```python
from build123d import *

# Parameters (mm, degrees)
SKETCH1_W   = 2.7
SKETCH1_H   = 10.5
SKETCH1_H_2 = 10.579195959
PANEL_DEPTH = 2.7


with BuildPart() as part:
    # Sketch1 → Panel (new body)
    with BuildSketch(Plane(origin=(0, 0, 0), x_dir=(0, 0, -1), z_dir=(1, 0, 0))):
        Polygon((3.2125, 30.5), (83.4125, 30.5), (94.9125, 30.5), (94.9125, -12.68), (86.975, -12.68), (6.775, -12.68), (-1.1625, -12.68), (-1.1625, 30.5), align=None)
        with Locations((8.125, 15.172642531)):
            Rectangle(SKETCH1_W, SKETCH1_H, mode=Mode.SUBTRACT)
        with Locations((85.625, 15.212240511)):
            Rectangle(SKETCH1_W, SKETCH1_H_2, mode=Mode.SUBTRACT)
        with Locations((28.125, 15.212240511)):
            Rectangle(SKETCH1_W, SKETCH1_H_2, mode=Mode.SUBTRACT)
    extrude(amount=PANEL_DEPTH)


solid = part.part
```
Check sheet for the modelled part. Datum: model origin and axes. Units: mm. A direction names the side the tool comes from. Round coordinates to 2 decimals unless told otherwise and drop trailing zeros. Write each loop counter-clockwise with the first axis right and the second up, starting at its lowest first coordinate (ties: lowest second). Pieces come first, ordered by that corner, then holes. Notation, with made-up numbers: M -11,54.5 L 46,54.5 A26 ccw 46,87.5 Z; hole C 81.5,84 d7. An arc over 180 degrees is marked long. Write item = value, one per line. Start each with the question number.
1. Scan lines: line 1 (Z direction, x = 2.4, y = 14) (1 decimal); line 2 (Y direction, x = 0.3, z = -84.5). Record each from-to range of solid material in increasing order. Write a range as [from, to].
2. Gauge pin test, flat end, axial feed: pin 1 (1 mm diameter, centred on y = 17.5, z = -69.5, fed in from -X). Record the tip position at first contact, or that the pin passes through.
3. Section check B-B, the plane z = -8. Record the cut outline in (x, y).
4. Tool access check on faces 1 (the flat face through (1, 9.923, -28)), 2 (the flat face through (1, 30.5, -48)). Record the directions out of +Z, -Z, +X, -X, +Y, -Y that give a thin tool (end or side, any length) a straight path to the whole face; none if there is none.
5. Release check for a two-part mould opening along Z. For faces 3 (the flat face through (2.7, 9, -48)), 4 (the flat face through (1, 20.423, -8)), 5 (the flat face through (1, 9, 1.162)) record: pulls with the +Z half, pulls with the -Z half, needs draft (parallel to the pull), parting line crosses it, or undercut.
6. Section check A-A, the plane y = 14. Record the cut outline in (x, z) (1 decimal), then the cut area to 3 significant figures.
7. Section check C-C, the plane x = 0.45. Record the cut outline in (y, z) (1 decimal).
Results found:
q1.line_1 = [-94.9, -87], [-84.3, -29.5], [-26.8, -9.5], [-6.8, 1.2]
q1.line_2 = [-12.68, 9.92], [20.5, 30.5]
q2.pin_1 = 0
q3.outline = M 0,-12.68 L 2.7,-12.68 L 2.7,9.92 L 0,9.92 Z; M 0,20.42 L 2.7,20.42 L 2.7,30.5 L 0,30.5 Z
q4.face_1 = +X, -X
q4.face_2 = +Z, -Z, +X, -X, +Y
q5.face_3 = needs draft
q5.face_4 = undercut
q5.face_5 = pulls with the +Z half
q6.outline = M 0,-94.9 L 2.7,-94.9 L 2.7,-87 L 0,-87 Z; M 0,-84.3 L 2.7,-84.3 L 2.7,-29.5 L 0,-29.5 Z; M 0,-26.8 L 2.7,-26.8 L 2.7,-9.5 L 0,-9.5 Z; M 0,-6.8 L 2.7,-6.8 L 2.7,1.2 L 0,1.2 Z
q6.area = 238 mm^2
q7.outline = M -12.7,-94.9 L 30.5,-94.9 L 30.5,1.2 L -12.7,1.2 Z; hole M 9.9,-87 L 20.5,-87 L 20.5,-84.3 L 9.9,-84.3 Z; hole M 9.9,-29.5 L 20.5,-29.5 L 20.5,-26.8 L 9.9,-26.8 Z; hole M 9.9,-9.5 L 20.4,-9.5 L 20.4,-6.8 L 9.9,-6.8 Z
